from build123d import *

# Parameters (mm, degrees)
EXTRUDE_1_DEPTH        = 40
SKETCH_3_R             = 1.75
SKETCH_3_R_2           = 28.55
MOTOR_FIXED_HOLE_DEPTH = 4
SKETCH_4_R             = 2.15
BASE_HOLE_DEPTH        = 4
FILLET_1_R             = 10


with BuildPart() as part:
    # 草圖2 → 填料-伸長1 (new body, symmetric)
    with BuildSketch(Plane(origin=(0, 0, 0), x_dir=(0, 0, -1), z_dir=(1, 0, 0))):
        Polygon((0, 80), (0, 0), (40, 0), (40, 3), (3, 3), (3, 80), align=None)
    extrude(amount=EXTRUDE_1_DEPTH, both=True)

    # 草圖3 → motor_fixed_hole (cut, through all)
    with BuildSketch(Plane(origin=(0, 0, -3), x_dir=(-1, 0, 0), z_dir=(0, 0, -1))):
        with Locations((17, 72.444863729)):
            Circle(SKETCH_3_R)
        with Locations((34, 43)):
            Circle(SKETCH_3_R)
        with Locations((17, 13.555136271)):
            Circle(SKETCH_3_R)
        with Locations((-17, 13.555136271)):
            Circle(SKETCH_3_R)
        with Locations((-34, 43)):
            Circle(SKETCH_3_R)
        with Locations((-17, 72.444863729)):
            Circle(SKETCH_3_R)
        with Locations((0, 43)):
            Circle(SKETCH_3_R_2)
    extrude(amount=-MOTOR_FIXED_HOLE_DEPTH, mode=Mode.SUBTRACT)

    # 草圖4 → base_hole (cut, through all)
    with BuildSketch(Plane(origin=(0, 3, 0), x_dir=(1, 0, 0), z_dir=(0, 1, 0))):
        with Locations((-30, 31.5)):
            Circle(SKETCH_4_R)
        with Locations((-30, 11.5)):
            Circle(SKETCH_4_R)
        with Locations((30, 11.5)):
            Circle(SKETCH_4_R)
        with Locations((30, 31.5)):
            Circle(SKETCH_4_R)
    extrude(amount=-BASE_HOLE_DEPTH, mode=Mode.SUBTRACT)

    # 圓角1
    fillet_1_edges = [part.edges().sort_by_distance(p)[0] for p in [
        (40, 1.5, -40),
        (40, 80, -1.5),
        (-40, 80, -1.5),
        (-40, 1.5, -40),
    ]]
    fillet(fillet_1_edges, radius=FILLET_1_R)


solid = part.part
Work out the finished part from the listing and answer in its coordinate system (mm). A direction names the side the tool comes from. Give positions to 0.01 mm unless a question says otherwise; leave off trailing zeros. Order: outer loops, then holes, each group sorted by start corner. A loop starts at its lowest first (then second) coordinate and runs counter-clockwise, first axis right, second up. Notation, with made-up numbers: (73, 62) -> (105, 62) arc R20 cw to (105, 67) -> close; hole circle Ø6 at (58, 49). An arc over 180 degrees is marked (long way). One line per item, written item: value.
Item 1: Find section A-A, the plane x = -10.5. Give the vertices of the cut face in (y, z).
Answer sheet:
outline: (0, -40) -> (3, -40) -> (3, -3) -> (16.45, -3) -> (16.45, 0) -> (0, 0) -> close; (69.55, -3) -> (80, -3) -> (80, 0) -> (69.55, 0) -> close
Item 2: Find section D-D, the plane x = 17. Give the vertices of the cut face in (y, z).
Answer sheet:
outline: (0, -40) -> (3, -40) -> (3, -3) -> (11.81, -3) -> (11.81, 0) -> (0, 0) -> close; (15.31, -3) -> (20.06, -3) -> (20.06, 0) -> (15.31, 0) -> close; (65.94, -3) -> (70.69, -3) -> (70.69, 0) -> (65.94, 0) -> close; (74.19, -3) -> (80, -3) -> (80, 0) -> (74.19, 0) -> close
Item 3: A tool of negligible diameter and unlimited length cuts with its end or side. For faces 1 (the flat face through (1, 0, -20)), 2 (the flat face through (9, 15, -3)), from which of +Z, -Z, +X, -X, +Y, -Y can it reach the whole face along a straight path? Write none if from no direction.
Answer sheet:
face 1: +Z, -Z, +X, -X, -Y
face 2: -Z, +X, -X, +Y
Item 4: Flat-ended cylindrical pins translate along their axes: P1, Ø8, axis at x = -15, z = -19.5, coming from the -Y side; P2, Ø3, axis at x = -27, y = 47, coming from the -Z side; P3, Ø2, axis at x = 26, z = -20.5, coming from the +Y side. Find the tip coordinate at first contact, or state that the pin passes through.
Answer sheet:
P1: y = 0
P2: z = -3
P3: y = 3
Item 5: Determine the mould class of faces 3 (the cylindrical face through (-33.62, 41.29, -1.52)), 4 (the cylindrical face through (31.16, 1.52, -33.31)), 5 (the cylindrical face through (37.15, 1.52, -36.99)), 6 (the flat face through (1, 3, -22)) for opening direction X: released by +X, released by -X, zero draft, split by the parting line, or undercut.
Answer sheet:
face 3: undercut
face 4: undercut
face 5: released by +X
face 6: zero draft
Item 6: Straight lines are drawn through the part: probe 1 along X at (y, z) = (1.6, -11.5); probe 2 along Z at (x, y) = (-30, 1.35); probe 3 along Y at (x, z) = (17, -1). For each, find the intervals that lie inside material, in ascending order.
Answer sheet:
probe 1: -40 to -32.15, -27.85 to 27.85, 32.15 to 40
probe 2: -40 to -33.65, -29.35 to -13.65, -9.35 to 0
probe 3: 0 to 11.81, 15.31 to 20.06, 65.94 to 70.69, 74.19 to 80
Item 7: Find section C-C, the plane y = 62. Give the vertices of the cut face in (x, z), plus the area to 3 significant figures.
Answer sheet:
outline: (-40, -3) -> (-21.31, -3) -> (-21.31, 0) -> (-40, 0) -> close; (21.31, -3) -> (40, -3) -> (40, 0) -> (21.31, 0) -> close
area: 112 mm²
Item 8: Find section B-B, the plane z = -11.5. Give the vertices of the cut face in (x, y).
Answer sheet:
outline: (-40, 0) -> (-32.15, 0) -> (-32.15, 3) -> (-40, 3) -> close; (-27.85, 0) -> (27.85, 0) -> (27.85, 3) -> (-27.85, 3) -> close; (32.15, 0) -> (40, 0) -> (40, 3) -> (32.15, 3) -> close
